Input: part model. Units: mm. Frame: model coordinates. Give positions to 0.01 mm unless a question says otherwise; leave off trailing zeros. Order: outer loops, then holes, each group sorted by start corner. A loop starts at its lowest first (then second) coordinate and runs counter-clockwise, first axis right, second up.
```python
from build123d import *

# Parameters (mm, degrees)
F0_W     = 62
F0_H     = 3.175
F1_DEPTH = 80
F3_D     = 4.4
F5_D     = 4.4
F4_R     = 27.5
F6_DEPTH = 25
F7_R     = 5


with BuildPart() as f1:
    # F0 (on Top) → F1 (new body)
    with BuildSketch(Plane.XY):
        Rectangle(F0_W, F0_H)
    extrude(amount=F1_DEPTH)

    # F3 (through all)
    with Locations(Plane(origin=(0, 1.5875, 0), x_dir=(-1, 0, 0), z_dir=(0, 1, 0))):
        with Locations((-6.5, 7.9375), (6.5, 7.9375)):
            Hole(F3_D / 2)

    # F5 (through all)
    with Locations(Plane(origin=(0, 1.5875, 0), x_dir=(-1, 0, 0), z_dir=(0, 1, 0))):
        with Locations((-25, 74), (25, 74), (25, 24), (-25, 24)):
            Hole(F5_D / 2)

    # F4 (on face) → F6 (cut)
    with BuildSketch(Plane(origin=(0, 1.5875, 0), x_dir=(-1, 0, 0), z_dir=(0, 1, 0))):
        with Locations((0, 49)):
            Circle(F4_R)
    extrude(amount=-F6_DEPTH, mode=Mode.SUBTRACT)

    # F7
    f7_edges = [f1.edges().sort_by_distance(p)[0] for p in [
        (31, 0, 80),
        (-31, 0, 80),
        (-31, 0, 0),
        (31, 0, 0),
    ]]
    fillet(f7_edges, radius=F7_R)


solid = f1.part
```
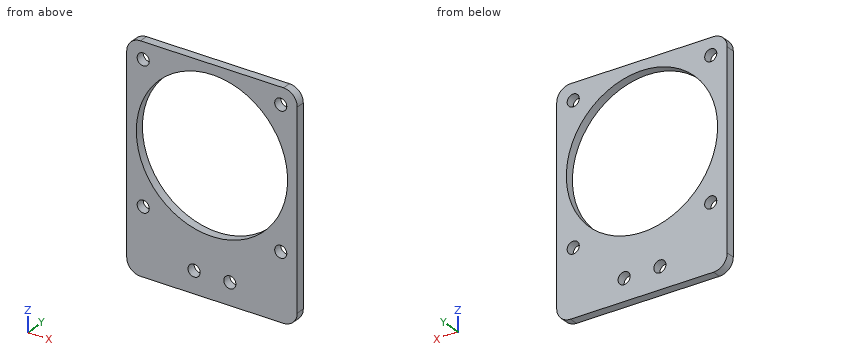
1) Cut plane D-D (z = 74). Return the cut outline in (x, y).
2) Cut plane C-C (x = 6.5). Return the cut outline in (y, z).
3) Cut plane A-A (x = -16.5). Return the cut outline in (y, z).
4) Cut plane B-B (z = 49). Return the cut outline in (x, y).
5) Line query: probe 1 along X at (y, z) = (-1.1, 8); probe 2 along Z at (x, y) = (0, -0.3); probe 3 along Z at (x, y) = (6.5, 0.65). Output: solid intervals per line, ascending.
Geometry says:
1. outline: (-31, -1.59) - (-27.2, -1.59) - (-27.2, 1.59) - (-31, 1.59) - close; (-22.8, -1.59) - (-11.46, -1.59) - (-11.46, 1.59) - (-22.8, 1.59) - close; (11.46, -1.59) - (22.8, -1.59) - (22.8, 1.59) - (11.46, 1.59) - close; (27.2, -1.59) - (31, -1.59) - (31, 1.59) - (27.2, 1.59) - close
2. outline: (-1.59, 0) - (1.59, 0) - (1.59, 5.74) - (-1.59, 5.74) - close; (-1.59, 10.14) - (1.59, 10.14) - (1.59, 22.28) - (-1.59, 22.28) - close; (-1.59, 75.72) - (1.59, 75.72) - (1.59, 80) - (-1.59, 80) - close
3. outline: (-1.59, 0) - (1.59, 0) - (1.59, 27) - (-1.59, 27) - close; (-1.59, 71) - (1.59, 71) - (1.59, 80) - (-1.59, 80) - close
4. outline: (-31, -1.59) - (-27.5, -1.59) - (-27.5, 1.59) - (-31, 1.59) - close; (27.5, -1.59) - (31, -1.59) - (31, 1.59) - (27.5, 1.59) - close
5. probe 1: x = -31 to -8.7, -4.3 to 4.3, 8.7 to 31
5. probe 2: z = 0 to 21.5, 76.5 to 80
5. probe 3: z = 0 to 5.74, 10.14 to 22.28, 75.72 to 80
